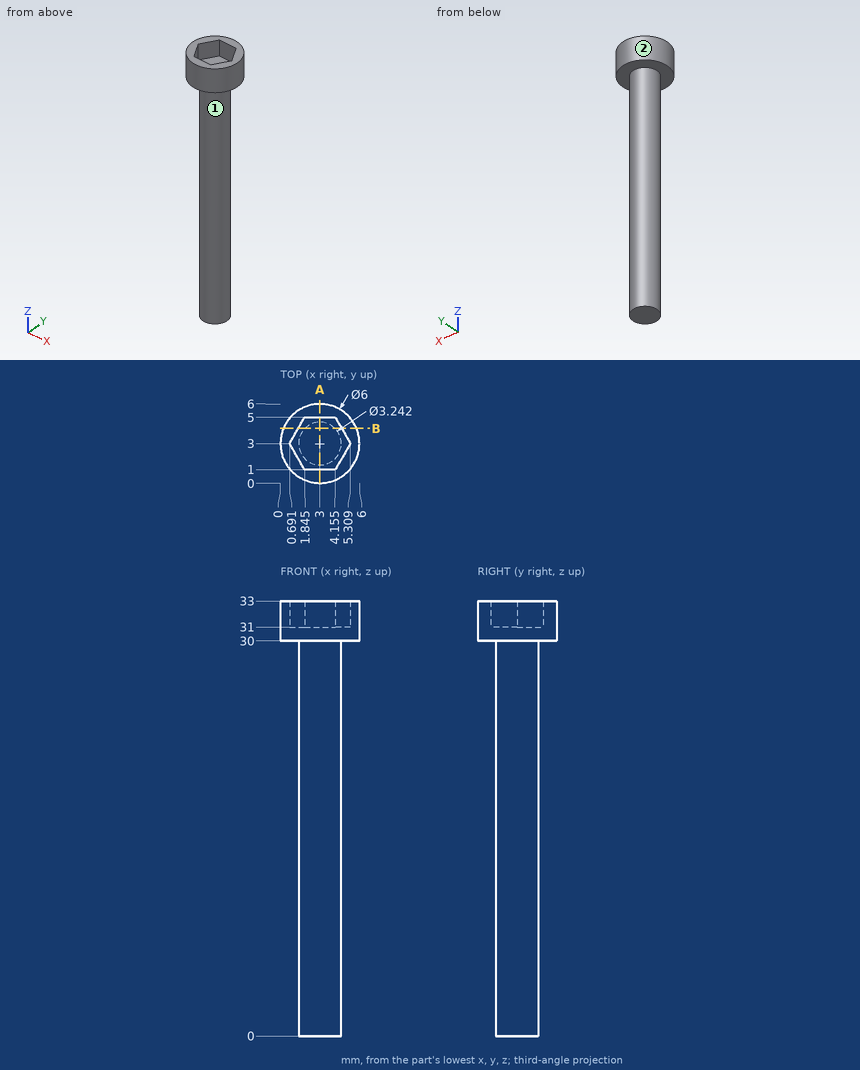
Answer from the drawing. Dimensions are ordinates in mm from the lowest x, y and z of the part. A direction names the side the tool comes from. Coordinates: 2 decimals unless noted, no trailing zeros. Write each loop counter-clockwise with the first axis right and the second up, starting at its lowest first coordinate (ties: lowest second). Pieces come first, ordered by that corner, then holes. Notation, with made-up numbers: M 3,-22.75 L 8,-22.75 A24 ccw 8,-2.75 Z; hole C -23.75,53.25 d8. An arc over 180 degrees is marked long. Write item = value, one per line.
1. The part is cut by section B-B (y = 4.15). Determine the outline of the cut face in (x, z) (1 decimal).
Solution:
outline = M 0.2,30 L 1.9,30 L 1.9,0 L 4.1,0 L 4.1,30 L 5.8,30 L 5.8,33 L 4.6,33 L 4.6,31 L 1.4,31 L 1.4,33 L 0.2,33 Z
2. The part is cut by section A-A (x = 3). Determine the outline of the cut face in (y, z).
Solution:
outline = M 0,30 L 1.38,30 L 1.38,0 L 4.62,0 L 4.62,30 L 6,30 L 6,33 L 5,33 L 5,31 L 1,31 L 1,33 L 0,33 Z
3. For the marked faces 1 and 2, determine the directions among +Z, -Z, +X, -X, +Y, -Y from which every point of the face is accessible in a straight line to the end or side of a thin tool.
Solution:
face_1 = -Z
face_2 = +Z, -Z
4. Straight lines are drawn through the part: line 1 (Z direction, x = 1.15, y = 2.95); line 2 (Z direction, x = 2.2, y = 3.35); line 3 (X direction, y = 2.85, z = 4) (1 decimal). For each, find the intervals that lie inside material, in ascending order. Write a range as from..to.
Solution:
line_1 = 30..31
line_2 = 0..31
line_3 = 1.4..4.6
5. Flat-ended cylindrical pins translate along their axes: pin 1 (1.5 mm diameter, centred on x = 3, z = 7.5, fed in from +Y); pin 2 (1 mm diameter, centred on x = 4.5, z = 12.5, fed in from +Y) (1 decimal). Find the tip coordinate at first contact, or state that the pin passes through.
Solution:
pin_1 = 4.62
pin_2 = 4.3
